Could you check a few things on this model? Use its own coordinates, in mm. A direction names the side the tool comes from. Round coordinates to 2 decimals unless told otherwise and drop trailing zeros. Write each loop counter-clockwise with the first axis right and the second up, starting at its lowest first coordinate (ties: lowest second). Pieces come first, ordered by that corner, then holes. Notation, with made-up numbers: (-27, 83) -> (20, 83) arc R10 cw to (20, 97) -> close; hole circle Ø7 at (36, 28). An arc over 180 degrees is marked (long way). Return JSON: item names as keys, results as strings.
from build123d import *

# Parameters (mm, degrees)
EXTRUDE_1_DEPTH     = 23
SKETCH_1_3_R        = 2.5
EXTRUDE_2_DEPTH     = 23
SKETCH_1_4_R        = 11
SKETCH_1_4_R_2      = 2.5
EXTRUDE_3_DEPTH     = 2
CUT_EXTRUDE_1_DEPTH = 10
SKETCH_2_W          = 32
SKETCH_2_H          = 7.5432644
CUT_EXTRUDE_2_DEPTH = 0.5
SKETCH_9_W          = 7.071067812
SKETCH_9_H          = 7.5432644
CUT_EXTRUDE_3_DEPTH = 0.5
SKETCH_8_W          = 32
SKETCH_8_H          = 7.5432644
CUT_EXTRUDE_4_DEPTH = 0.5
SKETCH_7_W          = 7.071067812
SKETCH_7_H          = 7.5432644
CUT_EXTRUDE_5_DEPTH = 0.5
SKETCH_6_W          = 32
SKETCH_6_H          = 7.5432644
CUT_EXTRUDE_6_DEPTH = 0.5
SKETCH_5_W          = 7.071067812
SKETCH_5_H          = 7.5432644
CUT_EXTRUDE_7_DEPTH = 0.5
SKETCH_4_W          = 32
SKETCH_4_H          = 7.5432644
CUT_EXTRUDE_8_DEPTH = 0.5
SKETCH_3_W          = 7.071067812
SKETCH_3_H          = 7.5432644
CUT_EXTRUDE_9_DEPTH = 0.5


with BuildPart() as part:
    # Sketch 1 → Extrude 1 (new body)
    with BuildSketch(Plane(origin=(0, 0, 0), x_dir=(1, 0, 0), z_dir=(0, 1, 0))):
        Polygon((-21, -16), (-16, -21), (16, -21), (21, -16), (21, 16), (16, 21), (-16, 21), (-21, 16), align=None)
    extrude(amount=-EXTRUDE_1_DEPTH)

    # Sketch 1_3 → Extrude 2 (add)
    with BuildSketch(Plane(origin=(0, 0, 0), x_dir=(1, 0, 0), z_dir=(0, 1, 0))):
        with Locations(Location((0, 0, 0), (0, 0, 270))):
            Circle(SKETCH_1_3_R)
    extrude(amount=EXTRUDE_2_DEPTH)

    # Sketch 1_4 → Extrude 3 (add)
    with BuildSketch(Plane(origin=(0, 0, 0), x_dir=(1, 0, 0), z_dir=(0, 1, 0))):
        with Locations(Location((0, 0, 0), (0, 0, 270))):
            Circle(SKETCH_1_4_R)
        with Locations(Location((0, 0, 0), (0, 0, 270))):
            Circle(SKETCH_1_4_R_2, mode=Mode.SUBTRACT)
    extrude(amount=EXTRUDE_3_DEPTH)

    # Sketch 1_5 → Cut-Extrude 1 (cut)
    with BuildSketch(Plane(origin=(0, 0, 0), x_dir=(1, 0, 0), z_dir=(0, 1, 0))):
        with BuildLine():
            Line((-15.5, -14), (-15.5, -15.5))
            Line((-15.5, -15.5), (-14, -15.5))
            ThreePointArc((-14, -15.5), (-14.439339828, -14.439339828), (-15.5, -14))
        make_face()
        with BuildLine():
            Line((-14, -15.5), (-15.5, -15.5))
            Line((-15.5, -15.5), (-15.5, -14))
            ThreePointArc((-15.5, -14), (-16.560660172, -16.560660172), (-14, -15.5))
        make_face()
        with BuildLine():
            ThreePointArc((-14, 15.5), (-16.560660172, 16.560660172), (-15.5, 14))
            Line((-15.5, 14), (-15.5, 15.5))
            Line((-15.5, 15.5), (-14, 15.5))
        make_face()
        with BuildLine():
            Line((-15.5, 15.5), (-15.5, 14))
            ThreePointArc((-15.5, 14), (-14.439339828, 14.439339828), (-14, 15.5))
            Line((-14, 15.5), (-15.5, 15.5))
        make_face()
        with BuildLine():
            ThreePointArc((14, 15.5), (14.439339828, 14.439339828), (15.5, 14))
            Line((15.5, 14), (15.5, 15.5))
            Line((15.5, 15.5), (14, 15.5))
        make_face()
        with BuildLine():
            Line((15.5, 15.5), (15.5, 14))
            ThreePointArc((15.5, 14), (16.560660172, 14.439339828), (17, 15.5))
            ThreePointArc((17, 15.5), (15.5, 17), (14, 15.5))
            Line((14, 15.5), (15.5, 15.5))
        make_face()
        with BuildLine():
            ThreePointArc((15.5, -14), (14.439339828, -14.439339828), (14, -15.5))
            Line((14, -15.5), (15.5, -15.5))
            Line((15.5, -15.5), (15.5, -14))
        make_face()
        with BuildLine():
            Line((15.5, -15.5), (14, -15.5))
            ThreePointArc((14, -15.5), (15.5, -17), (17, -15.5))
            ThreePointArc((17, -15.5), (16.560660172, -14.439339828), (15.5, -14))
            Line((15.5, -14), (15.5, -15.5))
        make_face()
    extrude(amount=-CUT_EXTRUDE_1_DEPTH, mode=Mode.SUBTRACT)

    # Sketch 2 → Cut-Extrude 2 (cut)
    with BuildSketch(Plane(origin=(0, 0, -21), x_dir=(-1, 0, 0), z_dir=(0, 0, -1))):
        with Locations((0, -11.2283678)):
            Rectangle(SKETCH_2_W, SKETCH_2_H)
    extrude(amount=-CUT_EXTRUDE_2_DEPTH, mode=Mode.SUBTRACT)

    # Sketch 9 → Cut-Extrude 3 (cut)
    with BuildSketch(Plane(origin=(-18.5, 0, -18.5), x_dir=(-0.7071067811865458, 0, 0.7071067811865492), z_dir=(-0.7071067811865492, 0, -0.7071067811865458))):
        with Locations((0, -11.2283678)):
            Rectangle(SKETCH_9_W, SKETCH_9_H)
    extrude(amount=-CUT_EXTRUDE_3_DEPTH, mode=Mode.SUBTRACT)

    # Sketch 8 → Cut-Extrude 4 (cut)
    with BuildSketch(Plane.ZY.offset(21)):
        with Locations((0, -11.2283678)):
            Rectangle(SKETCH_8_W, SKETCH_8_H)
    extrude(amount=-CUT_EXTRUDE_4_DEPTH, mode=Mode.SUBTRACT)

    # Sketch 7 → Cut-Extrude 5 (cut)
    with BuildSketch(Plane(origin=(-18.5, 0, 18.5), x_dir=(0.7071067811865475, 0, 0.7071067811865477), z_dir=(-0.7071067811865477, 0, 0.7071067811865475))):
        with Locations((0, -11.2283678)):
            Rectangle(SKETCH_7_W, SKETCH_7_H)
    extrude(amount=-CUT_EXTRUDE_5_DEPTH, mode=Mode.SUBTRACT)

    # Sketch 6 → Cut-Extrude 6 (cut)
    with BuildSketch(Plane.XY.offset(21)):
        with Locations((0, -11.2283678)):
            Rectangle(SKETCH_6_W, SKETCH_6_H)
    extrude(amount=-CUT_EXTRUDE_6_DEPTH, mode=Mode.SUBTRACT)

    # Sketch 5 → Cut-Extrude 7 (cut)
    with BuildSketch(Plane(origin=(18.5, 0, 18.5), x_dir=(0.7071067811865483, 0, -0.7071067811865468), z_dir=(0.7071067811865468, 0, 0.7071067811865483))):
        with Locations((0, -11.2283678)):
            Rectangle(SKETCH_5_W, SKETCH_5_H)
    extrude(amount=-CUT_EXTRUDE_7_DEPTH, mode=Mode.SUBTRACT)

    # Sketch 4 → Cut-Extrude 8 (cut)
    with BuildSketch(Plane(origin=(21, 0, 0), x_dir=(0, 0, -1), z_dir=(1, 0, 0))):
        with Locations((0, -11.2283678)):
            Rectangle(SKETCH_4_W, SKETCH_4_H)
    extrude(amount=-CUT_EXTRUDE_8_DEPTH, mode=Mode.SUBTRACT)

    # Sketch 3 → Cut-Extrude 9 (cut)
    with BuildSketch(Plane(origin=(18.5, 0, -18.5), x_dir=(-0.7071067811865483, 0, -0.7071067811865468), z_dir=(0.7071067811865468, 0, -0.7071067811865483))):
        with Locations((0, -11.2283678)):
            Rectangle(SKETCH_3_W, SKETCH_3_H)
    extrude(amount=-CUT_EXTRUDE_9_DEPTH, mode=Mode.SUBTRACT)


solid = part.part
1) I want a section at C-C, the plane x = 0. Please give me the cut outline in (y, z), and give its area (3 significant figures).
Return value:
{"outline": "(-23, -21) -> (-15, -21) -> (-15, -20.5) -> (-7.46, -20.5) -> (-7.46, -21) -> (0, -21) -> (0, -11) -> (2, -11) -> (2, -2.5) -> (23, -2.5) -> (23, 2.5) -> (2, 2.5) -> (2, 11) -> (0, 11) -> (0, 21) -> (-7.46, 21) -> (-7.46, 20.5) -> (-15, 20.5) -> (-15, 21) -> (-23, 21) -> close", "area": "1,110 mm²"}
2) I want a section at D-D, the plane z = -12. Please give me the cut outline in (x, y), and give its area (3 significant figures).
Return value:
{"outline": "(-21, -23) -> (21, -23) -> (21, -15) -> (20.5, -15) -> (20.5, -7.46) -> (21, -7.46) -> (21, 0) -> (-21, 0) -> (-21, -7.46) -> (-20.5, -7.46) -> (-20.5, -15) -> (-21, -15) -> close", "area": "958 mm²"}
3) I want a section at B-B, the plane z = 0. Please give me the cut outline in (x, y).
Return value:
{"outline": "(-21, -23) -> (21, -23) -> (21, -15) -> (20.5, -15) -> (20.5, -7.46) -> (21, -7.46) -> (21, 0) -> (11, 0) -> (11, 2) -> (2.5, 2) -> (2.5, 23) -> (-2.5, 23) -> (-2.5, 2) -> (-11, 2) -> (-11, 0) -> (-21, 0) -> (-21, -7.46) -> (-20.5, -7.46) -> (-20.5, -15) -> (-21, -15) -> close"}
4) Thinking about a two-plate mould opening in Y: for faces 5 (the face through (-20.5, -11, 0)), 6 (the face through (-21, -19, 0)), 7 (the face through (0, 23, 0)), which applies, pulls with the +Y half, pulls with the -Y half, needs draft (parallel to the pull), parting line crosses it, or undercut?
Return value:
{"face 5": "undercut", "face 6": "needs draft", "face 7": "pulls with the +Y half"}
5) If I drill on probe 1 along Z at (x, y) = (-15.5, -6.5); probe 2 along Z at (x, y) = (-15.5, -7.75), over which ranges is the centre line in solid material (lowest first)? Write a range as [from, to].
Return value:
{"probe 1": "[-21, -17], [-14, 14], [17, 21]", "probe 2": "[-20.5, -17], [-14, 14], [17, 20.5]"}
6) I want a section at A-A, the plane y = -9. Please give me the cut outline in (x, z).
Return value:
{"outline": "(-20.5, -15.79) -> (-15.79, -20.5) -> (15.79, -20.5) -> (20.5, -15.79) -> (20.5, 15.79) -> (15.79, 20.5) -> (-15.79, 20.5) -> (-20.5, 15.79) -> close; hole circle Ø3 at (-15.5, -15.5); hole circle Ø3 at (-15.5, 15.5); hole circle Ø3 at (15.5, -15.5); hole circle Ø3 at (15.5, 15.5)"}
7) For faces 1 (the face through (20.5, -11, 0)), 2 (the face through (-10.74, 0.99, -2.38)), 3 (the face through (0, -23, 0)), 4 (the face through (18.179, -11.176, -18.113)), which set-ups out of +Z, -Z, +X, -X, +Y, -Y let a thin tool reach every point of the face, with its end or its side?
Return value:
{"face 1": "+Z, -Z, +X", "face 2": "+Y", "face 3": "+Z, -Z, +X, -X, -Y", "face 4": "-Z, +X"}
8) Will these pins go through, and if not, where does the flat tip stop? pin 1 Ø2.5 at (x, z) = (-15.5, 15.5) entering from +Y; pin 2 Ø4 at (x, z) = (-4, -4.5) entering from +Y; pin 3 Ø1 at (x, y) = (-0.5, 3) entering from +Z.
Return value:
{"pin 1": "y = -10", "pin 2": "y = 2", "pin 3": "z = 2.5"}
